Model file for the job. Use its own axes, mm. Round coordinates to 2 decimals unless told otherwise and drop trailing zeros. Order: outer loops, then holes, each group sorted by start corner. A loop starts at its lowest first (then second) coordinate and runs counter-clockwise, first axis right, second up. Notation, with made-up numbers: (30.5, 17) -> (84.5, 17) arc R34 cw to (84.5, 55) -> close; hole circle Ø2 at (-14.5, 8.5). An arc over 180 degrees is marked (long way). Use CSV: the item, a comma, the result in double quotes.
```python
from build123d import *

# Parameters (mm, degrees)
SKETCH2_R           = 11.1125
BOSS_EXTRUDE1_DEPTH = 3.175


with BuildPart() as part:
    # Sketch2 → Boss-Extrude1 (new body)
    with BuildSketch(Plane(origin=(0, 0, 0), x_dir=(0, 0, -1), z_dir=(1, 0, 0))):
        with BuildLine():
            Line((13.719623131, 3.988056845), (-6.809679404, 74.6125))
            Line((-6.809679404, 74.6125), (-73.341598004, 74.6125))
            Line((-73.341598004, 74.6125), (-73.341598004, 23.8125))
            Line((-73.341598004, 23.8125), (-63.081952462, 17.823474758))
            Line((-63.081952462, 17.823474758), (-7.202854458, -12.339025242))
            ThreePointArc((-7.202854458, -12.339025242), (8.789793561, -11.263755386), (13.719623131, 3.988056845))
        make_face()
        with Locations((-55.879098004, 30.1625)):
            Circle(SKETCH2_R, mode=Mode.SUBTRACT)
        Circle(SKETCH2_R, mode=Mode.SUBTRACT)
    extrude(amount=BOSS_EXTRUDE1_DEPTH)


solid = part.part
```
Q1. Mould opens along Y. For faces 1 (the flat face through (1.57, 20.86, 68.28)), 2 (the flat face through (2, 74.612, 40)), 3 (the cylindrical face through (1.57, 3.34, -10.6)) say: +Y half, -Y half, draft (parallel to the pull), parting line (faces both ways), or undercut.
From the geometry:
face 1,"-Y half"
face 2,"+Y half"
face 3,"undercut"
Q2. Pin check, flat tips, straight feed: pin 1 (1 mm diameter, centred on x = 1.5, z = 54.5, fed in from -Y); pin 2 (4 mm diameter, centred on y = 15.5, z = -1, fed in from -X). Stop position of each tip, or through.
From the geometry:
pin 1,"stops at y = 12.92"
pin 2,"stops at x = 0"
Q3. Cut at B-B (y = 0). Give the cut face in (x, z) (1 decimal), plus the area to 3 significant figures.
From the geometry:
outline,"(0, -14.3) -> (3.2, -14.3) -> (3.2, -11.1) -> (0, -11.1) -> close; (0, 11.1) -> (3.2, 11.1) -> (3.2, 30.1) -> (0, 30.1) -> close"
area,"70.2 mm²"
Q4. Cut at C-C (x = 2). Give the cut face in (y, z) (1 decimal), plus the area to 3 significant figures.
From the geometry:
outline,"(-12.3, 7.2) arc R14.3 ccw to (4, -13.7) -> (74.6, 6.8) -> (74.6, 73.3) -> (23.8, 73.3) -> (17.8, 63.1) -> close; hole circle Ø22.2 at (0, 0); hole circle Ø22.2 at (30.2, 55.9)"
area,"4,890 mm²"
Q5. Probe line 1 along Y through (x, z) = (2.5, 62); line 2 along Y through (x, z) = (1.25, 56); line 3 along Z through (x, y) = (0.85, 28.5). List the from-to ranges inside material, lowest first.
From the geometry:
line 1,"y = 17.24 to 20.89, 39.44 to 74.61"
line 2,"y = 14 to 19.05, 41.27 to 74.61"
line 3,"z = -6.59 to 44.89, 66.87 to 73.34"
Q6. Cut at A-A (z = 0). Give the cut face in (x, y) (1 decimal).
From the geometry:
outline,"(0, -14.3) -> (3.2, -14.3) -> (3.2, -11.1) -> (0, -11.1) -> close; (0, 11.1) -> (3.2, 11.1) -> (3.2, 51.2) -> (0, 51.2) -> close"
Q7. Cut at D-D (y = 51). Give the cut face in (x, z) (3 decimals).
From the geometry:
outline,"(0, -0.054) -> (3.175, -0.054) -> (3.175, 73.342) -> (0, 73.342) -> close"
